Study the drawing (mm; zero at the part's minimum x, y, z) and answer. A direction names the side the tool comes from. Coordinates: 2 decimals unless noted, no trailing zeros. Order: outer loops, then holes, each group sorted by start corner. A loop starts at its lowest first (then second) coordinate and runs counter-clockwise, first axis right, second up. Notation, with made-up numbers: (4.25, 74) -> (41.25, 74) arc R13 cw to (41.25, 99) -> close; hole circle Ø5 at (45.25, -24.75). An arc over 180 degrees is marked (long way). One line per question, with ' | ' between items.
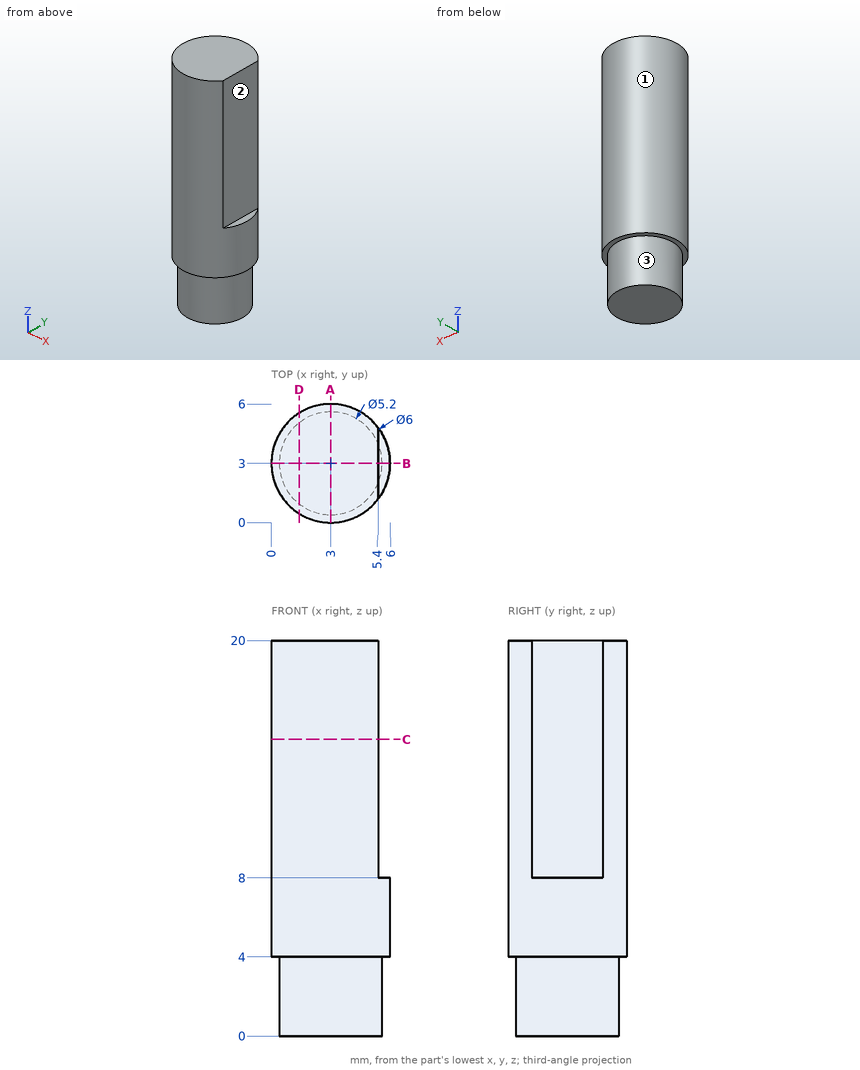
Item 1: Section C-C, the plane z = 15 is taken. Give the vertices of the cut face in (x, y).
Computed values:
outline: (5.4, 1.2) -> (5.4, 4.8) arc R3 ccw (long way) to start
Item 2: Section B-B, the plane y = 3 is taken. Give the vertices of the cut face in (x, z).
Computed values:
outline: (0, 4) -> (0.4, 4) -> (0.4, 0) -> (5.6, 0) -> (5.6, 4) -> (6, 4) -> (6, 8) -> (5.4, 8) -> (5.4, 20) -> (0, 20) -> close
Item 3: For the marked faces 1, 2 and 3, determine the directions among +Z, -Z, +X, -X, +Y, -Y from which every point of the face is accessible in a straight line to the end or side of a thin tool.
Computed values:
face 1: +Z, -Z | face 2: +Z, +X, +Y, -Y | face 3: -Z
Item 4: Section A-A, the plane x = 3 is taken. Give the vertices of the cut face in (y, z), plus the area to 3 significant figures.
Computed values:
outline: (0, 4) -> (0.4, 4) -> (0.4, 0) -> (5.6, 0) -> (5.6, 4) -> (6, 4) -> (6, 20) -> (0, 20) -> close | area: 117 mm^2
Item 5: Each of these flat-tipped pins is pushed along its axis until it touches: pin 1 Ø1.1 at (y, z) = (3, 16) entering from +X; pin 2 Ø1.5 at (x, z) = (4, 4) entering from -Y; pin 3 Ø1 at (y, z) = (2, 17.5) entering from -X. Where does it stop, or does it pass through?
Computed values:
pin 1: stops at x = 5.4 | pin 2: stops at y = 0.01 | pin 3: stops at x = 0.04
Item 6: Find the intervals of material crossed by L1, parallel to X at y = 2.9, z = 16; L2, parallel to Y at x = 2.85, z = 2; L3, parallel to Y at x = 5.4, z = 7.25, in increasing order.
Computed values:
L1: x = 0 to 5.4 | L2: y = 0.4 to 5.6 | L3: y = 1.2 to 4.8
Item 7: Section D-D, the plane x = 1.4 is taken. Give the vertices of the cut face in (y, z), plus the area to 3 significant figures.
Computed values:
outline: (0.46, 4) -> (0.95, 4) -> (0.95, 0) -> (5.05, 0) -> (5.05, 4) -> (5.54, 4) -> (5.54, 20) -> (0.46, 20) -> close | area: 97.6 mm^2
